```python
from build123d import *

# Parameters (mm, degrees)
SKETCH1_R               = 23.36
BOSS_EXTRUDE1_DEPTH     = 120
SHELL1_T                = -4
BOSS_EXTRUDE2_START     = -78
BOSS_EXTRUDE2_DEPTH     = 28
CUT_EXTRUDE2_START      = -3
SKETCH3_W               = 13.306682786
SKETCH3_H               = 112.078747136
CUT_EXTRUDE2_DEPTH      = 3
CIRPATTERN1_COUNT       = 6
CUT_EXTRUDE3_REACH      = 131.848
CUT_EXTRUDE3_END_RADIUS = 19.36
SKETCH4_R               = 1.7
CIRPATTERN2_COUNT       = 6


with BuildPart() as part:
    # Sketch1 → Boss-Extrude1 (new body)
    with BuildSketch(Plane(origin=(0, 0, 0), x_dir=(1, 0, 0), z_dir=(0, 1, 0))):
        with Locations(Location((0, 0, 0), (0, 0, 270))):
            Circle(SKETCH1_R)
    extrude(amount=BOSS_EXTRUDE1_DEPTH)

    # Shell1
    shell1_openings = [part.faces().sort_by_distance(p)[0] for p in [
        (0, 120, 0),
        (0, 0, 0),
    ]]
    offset(amount=SHELL1_T, openings=shell1_openings, kind=Kind.INTERSECTION)

    # Sketch2 → Boss-Extrude2 (add)
    with BuildSketch(Plane.XZ.offset(BOSS_EXTRUDE2_START)):
        with BuildLine():
            Line((-6.645158283, -18.183824444), (-5.892390902, -16.239003125))
            ThreePointArc((-5.892390902, -16.239003125), (-14.960585543, -8.63749809), (-17.00958469, 3.016541352))
            Line((-17.00958469, 3.016541352), (-19.070233048, 3.337036337))
            ThreePointArc((-19.070233048, 3.337036337), (-16.766251817, -9.68), (-6.645158283, -18.183824444))
        make_face()
        with BuildLine():
            ThreePointArc((17.00958469, 3.016541352), (14.960585543, -8.63749809), (5.892390902, -16.239003125))
            Line((5.892390902, -16.239003125), (6.645158283, -18.183824444))
            ThreePointArc((6.645158283, -18.183824444), (16.766251817, -9.68), (19.070233048, 3.337036337))
            Line((19.070233048, 3.337036337), (17.00958469, 3.016541352))
        make_face()
        with BuildLine():
            Line((-12.425074765, 14.846788107), (-11.117193788, 13.222461773))
            ThreePointArc((-11.117193788, 13.222461773), (0, 17.274996181), (11.117193788, 13.222461773))
            Line((11.117193788, 13.222461773), (12.425074765, 14.846788107))
            ThreePointArc((12.425074765, 14.846788107), (0, 19.36), (-12.425074765, 14.846788107))
        make_face()
    extrude(amount=BOSS_EXTRUDE2_DEPTH)

    # Sketch3 → Cut-Extrude2 (cut)
    with BuildSketch(Plane(origin=(0, 0, -26.4), x_dir=(-1, 0, 0), z_dir=(0, 0, -1)).offset(CUT_EXTRUDE2_START)):
        with Locations((0, 56.039373568)):
            Rectangle(SKETCH3_W, SKETCH3_H)
    cut_extrude2 = extrude(amount=-CUT_EXTRUDE2_DEPTH, mode=Mode.SUBTRACT)

    # CirPattern1: Cut-Extrude2 ×6 about axis
    cirpattern1_axis = Axis((0, 0, 0), (0, 1, 0))
    for i in range(1, CIRPATTERN1_COUNT):
        add(cut_extrude2.rotate(cirpattern1_axis, i * 360 / CIRPATTERN1_COUNT), mode=Mode.SUBTRACT)

    # Cut-Extrude3: up to this cylinder (the profile starts outside it)
    cut_extrude3_end = Plane(origin=(0, 60.2277495, 0), z_dir=(0, -1, 0)) * Cylinder(CUT_EXTRUDE3_END_RADIUS, 388.602281, mode=Mode.PRIVATE)
    # Sketch4 → Cut-Extrude3 (cut, up to the surface)
    with BuildSketch(Plane(origin=(0, 0, -20.4), x_dir=(-1, 0, 0), z_dir=(0, 0, -1)), mode=Mode.PRIVATE) as cut_extrude3_sk1:
        with Locations((0, 102.820889633)):
            Circle(SKETCH4_R)
    cut_extrude3_tool1 = extrude(cut_extrude3_sk1.sketch, amount=-CUT_EXTRUDE3_REACH, mode=Mode.PRIVATE) - cut_extrude3_end
    # Sketch4 → Cut-Extrude3 (cut, up to the surface)
    with BuildSketch(Plane(origin=(0, 0, -20.4), x_dir=(-1, 0, 0), z_dir=(0, 0, -1)), mode=Mode.PRIVATE) as cut_extrude3_sk2:
        with Locations((0, 17.634608904)):
            Circle(SKETCH4_R)
    cut_extrude3_tool2 = extrude(cut_extrude3_sk2.sketch, amount=-CUT_EXTRUDE3_REACH, mode=Mode.PRIVATE) - cut_extrude3_end
    cut_extrude3 = cut_extrude3_tool1.solids().sort_by_distance((0, 102.82089, -20.4))[0] + cut_extrude3_tool2.solids().sort_by_distance((0, 17.634609, -20.4))[0]
    add(cut_extrude3, mode=Mode.SUBTRACT)

    # CirPattern2: Cut-Extrude3 ×6 about axis
    cirpattern2_axis = Axis((0, 120, 0), (0, -1, 0))
    for i in range(1, CIRPATTERN2_COUNT):
        add(cut_extrude3.rotate(cirpattern2_axis, i * 360 / CIRPATTERN2_COUNT), mode=Mode.SUBTRACT)


solid = part.part
```
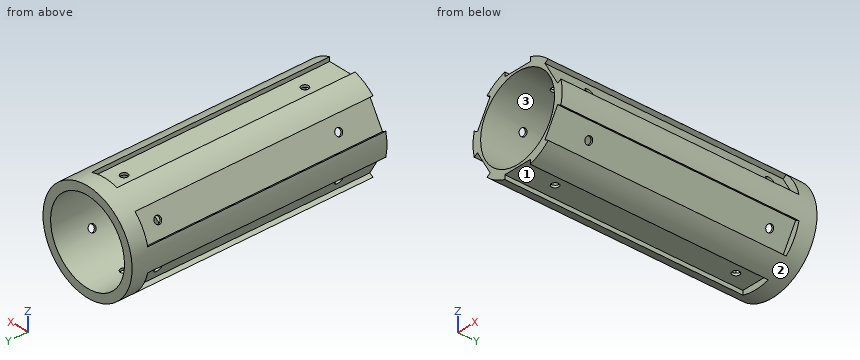
Part model, mm, in its own coordinate system. Face numbers are marked on the shaded views. Round coordinates to 2 decimals unless told otherwise and drop trailing zeros. Write each loop counter-clockwise with the first axis right and the second up, starting at its lowest first coordinate (ties: lowest second). Pieces come first, ordered by that corner, then holes.
Item 1: Two-plate mould, pull along X, no slides. Class the marked faces 1, 2 and 3: +X half, -X half, draft (parallel to the pull), parting line (faces both ways), or undercut.
Results:
face 1: undercut
face 2: parting line
face 3: undercut
Item 2: Probe L1, parallel to Y at x = 0, z = 19.6; L2, parallel to Z at x = 0, y = 41; L3, parallel to X at y = 6, z = -0.5. List the from-to ranges inside material, lowest first.
Results:
L1: y = 0 to 15.93, 19.33 to 101.12, 104.52 to 120
L2: z = -20.4 to -19.36, 19.36 to 20.4
L3: x = -23.35 to -19.35, 19.35 to 23.35
Item 3: Cut at A-A, the plane y = 46. Give the cut face in (x, z), plus the area to 3 significant figures.
Results:
outline: (-22.72, -5.43) - (-20.99, -4.44) - (-14.34, -15.96) - (-16.07, -16.96) arc R23.36 ccw to (-6.65, -22.39) - (-6.65, -20.4) - (6.65, -20.4) - (6.65, -22.39) arc R23.36 ccw to (16.07, -16.96) - (14.34, -15.96) - (20.99, -4.44) - (22.72, -5.43) arc R23.36 ccw to (22.72, 5.43) - (20.99, 4.44) - (14.34, 15.96) - (16.07, 16.96) arc R23.36 ccw to (6.65, 22.39) - (6.65, 20.4) - (-6.65, 20.4) - (-6.65, 22.39) arc R23.36 ccw to (-16.07, 16.96) - (-14.34, 15.96) - (-20.99, 4.44) - (-22.72, 5.43) arc R23.36 ccw to start; hole circle Ø38.72 at (0, 0)
area: 326 mm2
Item 4: Cut at C-C, the plane x = 0. Count the separate pieces of the cut face and the enclosed holes in it, plus the area to 3 significant figures.
Results:
separate pieces: 6
enclosed holes: 0
area: 341 mm2
Item 5: Drop flat-ended pins along their axis: pin 1 Ø1.6 at (y, z) = (59, -21) entering from -X; pin 2 Ø1.5 at (x, z) = (-1, 22.5) entering from -Y; pin 3 Ø2.5 at (x, y) = (0, 102.82) entering from +Z; pin 4 Ø2 at (y, z) = (74, 22) entering from -X. Give the stop position or say it passes through.
Results:
pin 1: stops at x = -11.73
pin 2: stops at y = 112.08
pin 3: passes through
pin 4: stops at x = -10.23
Item 6: Cut at B-B, the plane z = 0. Give the cut face in (x, y) (3 decimals), plus the area to 3 significant figures.
Results:
outline: (-23.36, 0) - (-19.36, 0) - (-19.36, 50) - (-17.275, 50) - (-17.275, 78) - (-19.36, 78) - (-19.36, 120) - (-23.36, 120) - close; (17.275, 50) - (19.36, 50) - (19.36, 0) - (23.36, 0) - (23.36, 120) - (19.36, 120) - (19.36, 78) - (17.275, 78) - close
area: 1,080 mm2
